Here's how the part is built. I have some questions about the finished solid (model axes, mm). Round coordinates to 2 decimals unless told otherwise and drop trailing zeros. Loops run counter-clockwise (first coordinate to the right, second up) from the corner with the lowest first, then second, coordinate; pieces in that order, holes last. Notation, with made-up numbers: M -31,80.5 L 7,80.5 A14 cw 7,88.5 Z; hole C 29.25,-40 d11. An arc over 180 degrees is marked long. Answer as a JSON object with one key per item and string values.
Autodesk Inventor part; units mm, degrees
ref_plane "YZ Plane" through (0, 0, 0) normal (1, 0, 0) x (0, 1, 0)
ref_plane "XZ Plane" through (0, 0, 0) normal (0, 1, 0) x (-1, 0, 0)
ref_plane "XY Plane" through (0, 0, 0) normal (0, 0, 1) x (1, 0, 0)
sketch "Sketch1" plane through (0, 0, 0) normal (0, 1, 0) x (-1, 0, 0)
  line L0 (-75, 100) -> (-55, 100)
  line L1 (-55, 100) -> (-55, 25)
  line L2 (-55, 25) -> (-75, 25)
  line L3 (-75, 25) -> (-75, -22)
  line L4 (-75, -22) -> (-55, -22)
  line L5 (-55, -22) -> (-55, -97)
  line L6 (-55, -97) -> (-75, -97)
  line L7 (0, 0) -> (0, -13.688)
  line L8 (0, 0) -> (16.407, 0)
  line L9 (75, 100) -> (55, 100)
  line L10 (55, 100) -> (55, 25)
  line L11 (55, 25) -> (75, 25)
  line L12 (75, 25) -> (75, -22)
  line L13 (75, -22) -> (55, -22)
  line L14 (55, -22) -> (55, -97)
  line L15 (55, -97) -> (75, -97)
  arc A0 (75, 100) -> (-75, 100) centre (0, 0) ccw
  arc A1 (-75, -97) -> (75, -97) centre (0, 3) ccw
  line L16 (-60, -3.5) -> (-65, -3.5)
  line L17 (-65, -3.5) -> (-65, 6.5)
  line L18 (-65, 6.5) -> (-60, 6.5)
  line L19 (-60, 6.5) -> (-60, -3.5)
  line L20 (60, -3.5) -> (65, -3.5)
  line L21 (65, -3.5) -> (65, 6.5)
  line L22 (65, 6.5) -> (60, 6.5)
  line L23 (60, 6.5) -> (60, -3.5)
extrude "Extrusion1" add sketch "Sketch1" along normal mid plane 3 contours A0 L9 L10 L11 L12 L13 L14 L15 A1 L6 L5 L4 L3 L2 L1 L0 | L16 L17 L18 L19 | L23 L22 L21 L20
sketch "Sketch2" plane through (0, 1.5, 0) normal (0, 1, 0) x (1, 0, 0)
  point P0 (0, 0)
sketch "Sketch3" plane through (0, 1.5, 0) normal (0, 1, 0) x (1, 0, 0)
  line L0 (65, 3.5) -> (60, 3.5)
  line L1 (60, 3.5) -> (60, -6.5)
  line L2 (60, -6.5) -> (65, -6.5)
  line L3 (65, -6.5) -> (65, 3.5)
  line L4 (0, 0) -> (0, -6.5)
  line L5 (-65, 3.5) -> (-60, 3.5)
  line L6 (-60, 3.5) -> (-60, -6.5)
  line L7 (-60, -6.5) -> (-65, -6.5)
  line L8 (-65, -6.5) -> (-65, 3.5)
extrude "Extrusion2" cut sketch "Sketch3" against normal blind 3 contours L3 L2 L1 L0
sketch "Sketch4" plane through (0, -1.5, 0) normal (0, -1, 0) x (1, 0, 0)
  line L0 (-60, -3.5) -> (-65, -3.5)
  line L1 (-65, -3.5) -> (-65, 6.5)
  line L2 (-65, 6.5) -> (-60, 6.5)
  line L3 (-60, 6.5) -> (-60, -3.5)
  point P0 (0, 0)
extrude "Extrusion3" cut sketch "Sketch4" against normal blind 3
sketch "Sketch5" plane through (0, -1.5, 0) normal (0, -1, 0) x (1, 0, 0)
  line L0 (-5, 110) -> (5, 110)
  line L1 (5, 110) -> (5, 115)
  line L2 (5, 115) -> (-5, 115)
  line L3 (-5, 115) -> (-5, 110)
  line L4 (0, 0) -> (8.5415, 0)
  line L5 (-5, -110) -> (5, -110)
  line L6 (5, -110) -> (5, -115)
  line L7 (5, -115) -> (-5, -115)
  line L8 (-5, -115) -> (-5, -110)
extrude "Extrusion4" cut sketch "Sketch5" against normal blind 3
sketch "Sketch6" plane through (0, -1.5, 0) normal (0, -1, 0) x (1, 0, 0)
  line L0 (-37.5, 72.5) -> (37.5, 72.5)
  line L1 (37.5, 72.5) -> (37.5, 52.5)
  line L2 (37.5, 52.5) -> (-37.5, 52.5)
  line L3 (-37.5, 52.5) -> (-37.5, 72.5)
  line L4 (0, 0) -> (15.5313, 0)
  line L5 (-37.5, -72.5) -> (37.5, -72.5)
  line L6 (37.5, -72.5) -> (37.5, -52.5)
  line L7 (37.5, -52.5) -> (-37.5, -52.5)
  line L8 (-37.5, -52.5) -> (-37.5, -72.5)
extrude "Extrusion5" cut sketch "Sketch6" against normal blind 3
sketch "Sketch7" plane through (0, -1.5, 0) normal (0, -1, 0) x (1, 0, 0)
  point P0 (0, 0)
sketch "Sketch8" plane through (0, -1.5, 0) normal (0, -1, 0) x (1, 0, 0)
  point P0 (0, 0)
properties part number "PakAnomRevisi"
Item 1: Please list where these lines run through material, in increasing order: probe 1 along Z at (x, y) = (0, -0.7); probe 2 along X at (y, z) = (-0.75, -64); probe 3 along Z at (x, y) = (24, 0.4). Write a range as from..to.
Resolved:
{"probe 1": "-122..-115, -110..-72.5, -52.5..52.5, 72.5..110, 115..125", "probe 2": "-55..-37.5, 37.5..55", "probe 3": "-119.67..-72.5, -52.5..52.5, 72.5..122.67"}
Item 2: I want a section at C-C, the plane y = 0.8. State how many separate pieces and enclosed holes the cut face has, then the cut area to 3 significant figures.
Resolved:
{"separate pieces": "1", "enclosed holes": "6", "area": "25,500 mm²"}
Item 3: I want a section at A-A, the plane x = -35. Please give me the cut outline in (y, z).
Resolved:
{"outline": "M -1.5,-117 L 1.5,-117 L 1.5,-72.5 L -1.5,-72.5 Z; M -1.5,-52.5 L 1.5,-52.5 L 1.5,52.5 L -1.5,52.5 Z; M -1.5,72.5 L 1.5,72.5 L 1.5,120 L -1.5,120 Z"}
Item 4: I want a section at D-D, the plane z = 80. Please give me the cut outline in (x, y).
Resolved:
{"outline": "M -55,-1.5 L 55,-1.5 L 55,1.5 L -55,1.5 Z"}
Item 5: I want a section at B-B, the plane x = -14.5. Please give me the cut outline in (y, z).
Resolved:
{"outline": "M -1.5,-121.16 L 1.5,-121.16 L 1.5,-72.5 L -1.5,-72.5 Z; M -1.5,-52.5 L 1.5,-52.5 L 1.5,52.5 L -1.5,52.5 Z; M -1.5,72.5 L 1.5,72.5 L 1.5,124.16 L -1.5,124.16 Z"}
Item 6: I'm going to push flat-ended pins straight in: pin 1 Ø0.9 at (x, y) = (62, 0) entering from -Z; pin 2 Ø1.5 at (y, z) = (-0.5, 66) entering from +X; pin 3 Ø0.9 at (y, z) = (0, -112) entering from -X. Where does each tip first touch, or does it pass through?
Resolved:
{"pin 1": "z = -105.8", "pin 2": "x = 55", "pin 3": "x = -50.03"}
